Geometry: final body of the model. Coordinates: model frame, mm. A direction names the side the tool comes from. Coordinates: 2 decimals unless noted, no trailing zeros. Write each loop counter-clockwise with the first axis right and the second up, starting at its lowest first coordinate (ties: lowest second). Pieces come first, ordered by that corner, then holes. Notation, with made-up numbers: (36.5, 33) -> (83.5, 33) arc R17 ccw to (83.5, 58) -> close; hole circle Ø9 at (73.5, 44). An arc over 180 degrees is marked (long way). One line per item, written item: value. Start each with the question number.
from build123d import *

# Parameters (mm, degrees)
SKETCH3_W           = 10
SKETCH3_H           = 10
BOSS_EXTRUDE3_DEPTH = 241
BOSS_EXTRUDE4_DEPTH = 5
FILLET1_R           = 3


with BuildPart() as part:
    # Sketch3 → Boss-Extrude3 (new body)
    with BuildSketch(Plane(origin=(0, 0, 0), x_dir=(1, 0, 0), z_dir=(0, 1, 0))):
        Rectangle(SKETCH3_W, SKETCH3_H)
    extrude(amount=BOSS_EXTRUDE3_DEPTH)

    # Sketch4 → Boss-Extrude4 (add)
    with BuildSketch(Plane.XY.offset(5)):
        with BuildLine():
            Line((5, 8.767157353), (5, 0))
            ThreePointArc((5, 0), (8.185559909, -2.404164639), (9.624006089, 1.318559113))
            Line((9.624006089, 1.318559113), (5, 8.767157353))
        make_face()
    extrude(amount=-BOSS_EXTRUDE4_DEPTH)

    # Fillet1
    fillet1_edges = [part.edges().sort_by_distance(p)[0] for p in [
        (-5, 120.5, -5),
        (5, 120.5, -5),
        (5, 124.883578677, 5),
        (-5, 120.5, 5),
    ]]
    fillet(fillet1_edges, radius=FILLET1_R)


solid = part.part
Q1. First-contact query: P1, Ø6, axis at x = 7, y = 207.5, coming from the -Z side; P2, Ø1.2, axis at y = 124.5, z = -0.5, coming from the +X side; P3, Ø5, axis at x = -3.5, z = -2, coming from the -Y side. Flat tips, straight axial feed; report the tip coordinate or a pass-through.
Q2. Access query for faces 1 (the flat face through (0, 0, 0)), 2 (the flat face through (0, 119, -5)), 3 (the flat face through (7, 2, 0)). Directions: +Z, -Z, +X, -X, +Y, -Y. A direction counts if a zero-diameter tool reaches every point of the face in a straight line with its end or side. Return the directions, or none.
Q3. Cut plane A-A on y = 198. Output: boundary loops of the cut face in (x, z).
Q4. Cut plane B-B on x = 7.5. Output: boundary loops of the cut face in (y, z).
Q5. Line query: L1, parallel to Y at x = 1.75, z = 0.75; L2, parallel to Z at x = -2.25, y = 84; L3, parallel to X at y = 78, z = -2.5. Output: solid intervals per line, ascending. Write a range as from..to.
Solution:
1. P1: z = -4.24
1. P2: x = 5
1. P3: y = 0
2. face 1: +Z, -Z, -X, -Y
2. face 2: -Z, +X, -X, +Y, -Y
2. face 3: -Z, +X, +Y, -Y
3. outline: (-5, -2) arc R3 ccw to (-2, -5) -> (2, -5) arc R3 ccw to (5, -2) -> (5, 2) arc R3 ccw to (2, 5) -> (-2, 5) arc R3 ccw to (-5, 2) -> close
4. outline: (-2.5, 0) -> (4.74, 0) -> (4.74, 5) -> (-2.5, 5) -> close
5. L1: 0..241
5. L2: -4.99..4.99
5. L3: -4.96..4.96
